Answer from the drawing. Dimensions are ordinates in mm from the lowest x, y and z of the part. A direction names the side the tool comes from. Round coordinates to 2 decimals unless told otherwise and drop trailing zeros. Order: outer loops, then holes, each group sorted by start corner. A loop starts at its lowest first (then second) coordinate and runs counter-clockwise, first axis right, second up.
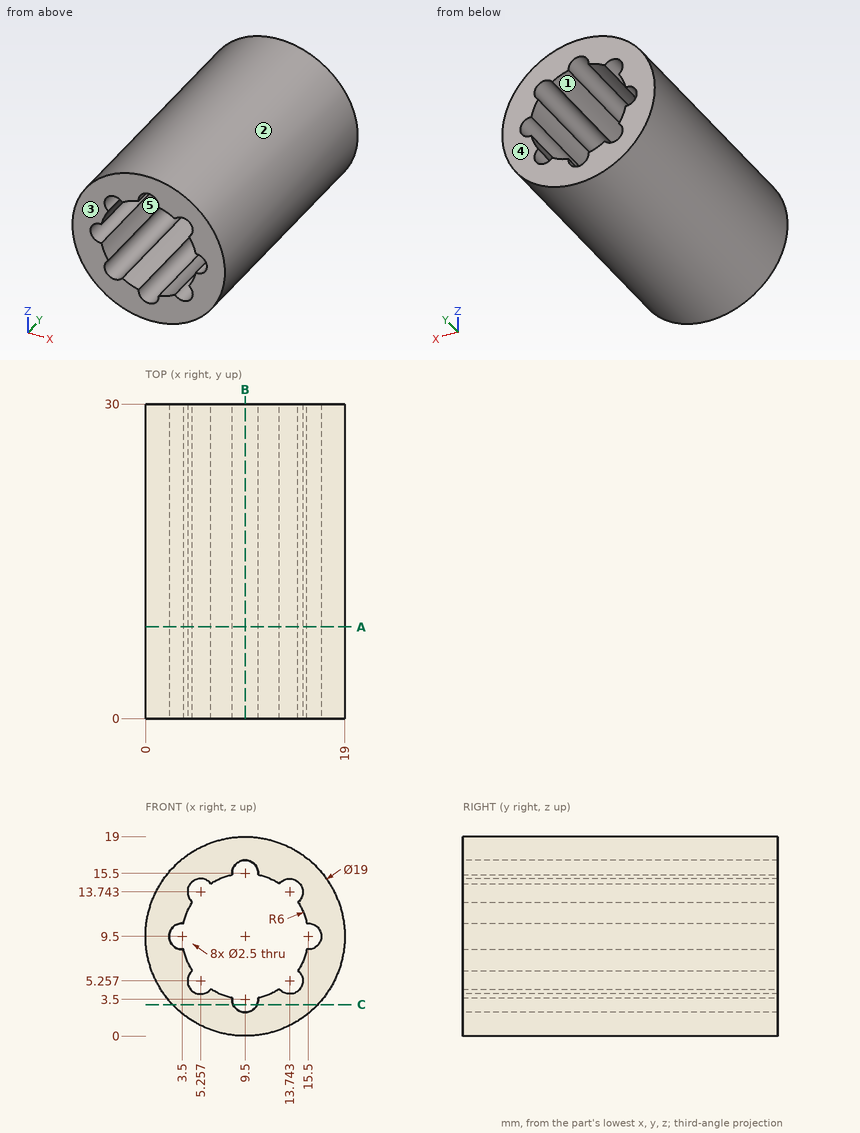
Q1. A cutting plane is placed at A-A, the plane y = 8.75. Give the vertices of the cut face in (x, z), plus the area to 3 significant figures.
Outcome:
outline: circle Ø19 at (9.5, 9.5); hole (3.63, 8.26) arc R6 ccw to (4.47, 6.23) arc R1.25 ccw (long way) to (6.23, 4.47) arc R6 ccw to (8.26, 3.63) arc R1.25 ccw (long way) to (10.74, 3.63) arc R6 ccw to (12.77, 4.47) arc R1.25 ccw (long way) to (14.53, 6.23) arc R6 ccw to (15.37, 8.26) arc R1.25 ccw (long way) to (15.37, 10.74) arc R6 ccw to (14.53, 12.77) arc R1.25 ccw (long way) to (12.77, 14.53) arc R6 ccw to (10.74, 15.37) arc R1.25 ccw (long way) to (8.26, 15.37) arc R6 ccw to (6.23, 14.53) arc R1.25 ccw (long way) to (4.47, 12.77) arc R6 ccw to (3.63, 10.74) arc R1.25 ccw (long way) to start
area: 150 mm2
Q2. For the marked faces 4 and 5, determine the directions among +Z, -Z, +X, -X, +Y, -Y from which every point of the face is accessible in a straight line to the end or side of a thin tool.
Outcome:
face 4: +Z, -Z, +X, -X, +Y
face 5: +Y, -Y
Q3. Flat-ended cylindrical pins translate along their axes: pin 1 (3 mm diameter, centred on y = 12.5, z = 13.5, fed in from -X) (1 decimal); pin 2 (2 mm diameter, centred on x = 13.74, z = 5.26, fed in from +Y) (1 decimal); pin 3 (2 mm diameter, centred on y = 11, z = 12.5, fed in from +X); pin 4 (3 mm diameter, centred on x = 16.5, y = 14, fed in from +Z) (1 decimal). Find the tip coordinate at first contact, or state that the pin passes through.
Outcome:
pin 1: stops at x = 0.3
pin 2: passes through
pin 3: stops at x = 18.79
pin 4: stops at z = 17.2
Q4. A cutting plane is placed at C-C, the plane z = 3. Give the vertices of the cut face in (x, y) (1 decimal).
Outcome:
outline: (2.6, 0) - (8.4, 0) - (8.4, 30) - (2.6, 30) - close; (10.6, 0) - (16.4, 0) - (16.4, 30) - (10.6, 30) - close
Q5. For a pull along X with two mould halves and no side action, classify the marked faces 1, 2 and 3 as released by +X, released by -X, zero draft, split by the parting line, or undercut.
Outcome:
face 1: undercut
face 2: split by the parting line
face 3: zero draft
Q6. Straight lines are drawn through the part: probe 1 along Z at (x, y) = (9.5, 11); probe 2 along Z at (x, y) = (8, 5); probe 3 along X at (y, z) = (8, 14) (1 decimal). For each, find the intervals that lie inside material, in ascending order.
Outcome:
probe 1: z = 0 to 2.25, 16.75 to 19
probe 2: z = 0.12 to 3.69, 15.31 to 18.88
probe 3: x = 1.1 to 4, 15 to 17.9
Q7. A cutting plane is placed at B-B, the plane x = 9.5. Give the vertices of the cut face in (y, z), plus the area to 3 significant figures.
Outcome:
outline: (0, 0) - (30, 0) - (30, 2.25) - (0, 2.25) - close; (0, 16.75) - (30, 16.75) - (30, 19) - (0, 19) - close
area: 135 mm2
